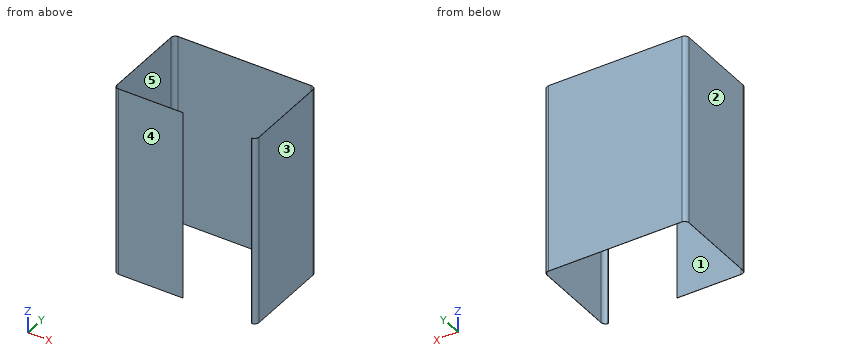
```python
from build123d import *

# Parameters (mm, degrees)
F1_DEPTH = 2200


with BuildPart() as f1:
    # F0 (on Top) → F1 (new body)
    with BuildSketch(Plane.XY):
        with BuildLine():
            ThreePointArc((825, 485), (810.355339, 520.355339), (775, 535))
            Line((775, 535), (-775, 535))
            ThreePointArc((-775, 535), (-810.355339, 520.355339), (-825, 485))
            Line((-825, 485), (-825, -485))
            ThreePointArc((-825, -485), (-810.355339, -520.355339), (-775, -535))
            Line((-775, -535), (-27, -535))
            Line((-27, -535), (-27, -533))
            Line((-27, -533), (-773, -533))
            ThreePointArc((-773, -533), (-808.355339, -518.355339), (-823, -483))
            Line((-823, -483), (-823, 483))
            ThreePointArc((-823, 483), (-808.355339, 518.355339), (-773, 533))
            Line((-773, 533), (773, 533))
            ThreePointArc((773, 533), (808.355339, 518.355339), (823, 483))
            Line((823, 483), (823, -483))
            ThreePointArc((823, -483), (808.355339, -518.355339), (773, -533))
            Line((773, -533), (772.985399, -535))
            Line((772.985399, -535), (775, -535))
            ThreePointArc((775, -535), (810.355339, -520.355339), (825, -485))
            Line((825, -485), (825, 485))
        make_face()
    extrude(amount=F1_DEPTH)


solid = f1.part
```
Input: part model. Units: mm. Frame: model coordinates. Face numbers are marked on the shaded views. A direction names the side the tool comes from. Round coordinates to 2 decimals unless told otherwise and drop trailing zeros. Write each loop counter-clockwise with the first axis right and the second up, starting at its lowest first coordinate (ties: lowest second). Pieces come first, ordered by that corner, then holes. Notation, with made-up numbers: (1.25, -24.5) -> (43.25, -24.5) arc R16 ccw to (43.25, -17.5) -> close; hole circle Ø10 at (38, 82). An arc over 180 degrees is marked (long way). Answer as CSV lines item,"result".
1. Section A-A (x = -473). Return the cut outline in (y, z).
Geometry says:
outline,"(-535, 0) -> (-533, 0) -> (-533, 2200) -> (-535, 2200) -> close; (533, 0) -> (535, 0) -> (535, 2200) -> (533, 2200) -> close"
2. Contact query for a flat-ended pin moving along its axis: P1, Ø8, axis at x = 26.5, z = 1507, coming from the -Y side. Output: stop coordinate, or through.
Geometry says:
P1,"stops at y = 533"
3. Section C-C (z = 1882). Return the cut outline in (x, y).
Geometry says:
outline,"(-825, -485) arc R50 ccw to (-775, -535) -> (-27, -535) -> (-27, -533) -> (-773, -533) arc R50 cw to (-823, -483) -> (-823, 483) arc R50 cw to (-773, 533) -> (773, 533) arc R50 cw to (823, 483) -> (823, -483) arc R50 cw to (773, -533) -> (772.99, -535) -> (775, -535) arc R50 ccw to (825, -485) -> (825, 485) arc R50 ccw to (775, 535) -> (-775, 535) arc R50 ccw to (-825, 485) -> close"
4. Ray query, L1, parallel to X at y = -201, z = 608.5; L2, parallel to Y at x = -288, z = 1376.5; L3, parallel to Y at x = 619.5, z = 360. Return the intervals inside material, ascending. Write a range as [from, to].
Geometry says:
L1,"x = [-825, -823], [823, 825]"
L2,"y = [-535, -533], [533, 535]"
L3,"y = [533, 535]"
5. Reachability of the marked faces 1 and 2 from +Z, -Z, +X, -X, +Y, -Y: full face, straight path, thin tool, end or side. Return the list, or none.
Geometry says:
face 1,"+Z, -Z"
face 2,"+Z, -Z, -X, +Y, -Y"
6. Mould query, pull axis Y, two halves, no side actions, for the marked faces 3, 4 and 5. Classes: +Y half, -Y half, draft (parallel to the pull), parting line (faces both ways), or undercut.
Geometry says:
face 3,"draft"
face 4,"-Y half"
face 5,"undercut"
7. Section D-D (x = 223). Return the cut outline in (y, z), plus the area to 3 significant figures.
Geometry says:
outline,"(533, 0) -> (535, 0) -> (535, 2200) -> (533, 2200) -> close"
area,"4,400 mm^2"
8. Section B-B (y = 451.5). Return the cut outline in (x, z).
Geometry says:
outline,"(-825, 0) -> (-823, 0) -> (-823, 2200) -> (-825, 2200) -> close; (823, 0) -> (825, 0) -> (825, 2200) -> (823, 2200) -> close"
